Could you check a few things on this model? Use its own coordinates, in mm. A direction names the side the tool comes from. Round coordinates to 2 decimals unless told otherwise and drop trailing zeros. Loops run counter-clockwise (first coordinate to the right, second up) from the corner with the lowest first, then second, coordinate; pieces in that order, holes last.
from build123d import *

# Parameters (mm, degrees)
BOSS_EXTRUDE1_DEPTH           = 13
BOSS_EXTRUDE1_OTHER_WAY_DEPTH = 13
BOSS_EXTRUDE1_OTHER_WAY_TAPER = -0.2
SKETCH3_R                     = 8.5
BOSS_EXTRUDE2_DEPTH           = 2
CUT_EXTRUDE2_DEPTH            = 12.5
SKETCH2_R                     = 1.25
CUT_EXTRUDE1_DEPTH            = 15
CUT_EXTRUDE3_DEPTH            = 15


with BuildPart() as part:
    # Sketch1 → Boss-Extrude1 (new body)
    with BuildSketch(Plane.XY):
        with BuildLine():
            ThreePointArc((-6.053717866, -0.75), (6.1, 0), (-6.053717866, 0.75))
            Line((-6.053717866, 0.75), (-6.853717866, 0.5))
            Line((-6.853717866, 0.5), (-6.853717866, -0.5))
            Line((-6.853717866, -0.5), (-6.053717866, -0.75))
        make_face()
    extrude(amount=BOSS_EXTRUDE1_DEPTH)

    # Sketch1 → Boss-Extrude1 other way (add)
    with BuildSketch(Plane.XY):
        with BuildLine():
            ThreePointArc((-6.053717866, -0.75), (6.1, 0), (-6.053717866, 0.75))
            Line((-6.053717866, 0.75), (-6.853717866, 0.5))
            Line((-6.853717866, 0.5), (-6.853717866, -0.5))
            Line((-6.853717866, -0.5), (-6.053717866, -0.75))
        make_face()
    extrude(amount=-BOSS_EXTRUDE1_OTHER_WAY_DEPTH, taper=BOSS_EXTRUDE1_OTHER_WAY_TAPER)

    # Sketch3 → Boss-Extrude2 (add)
    with BuildSketch(Plane(origin=(0, 0, -13), x_dir=(-1, 0, 0), z_dir=(0, 0, -1))):
        Circle(SKETCH3_R)
    extrude(amount=BOSS_EXTRUDE2_DEPTH)

    # Sketch4 → Cut-Extrude2 (cut)
    with BuildSketch(Plane(origin=(0, 0, -15), x_dir=(-1, 0, 0), z_dir=(0, 0, -1))):
        with BuildLine():
            Line((2.5, 1.833030278), (2.5, -1.833030278))
            ThreePointArc((2.5, -1.833030278), (-3.1, 0), (2.5, 1.833030278))
        make_face()
    extrude(amount=-CUT_EXTRUDE2_DEPTH, mode=Mode.SUBTRACT)

    # Sketch2 → Cut-Extrude1 (cut)
    with BuildSketch(Plane.XY.offset(13)):
        Circle(SKETCH2_R)
    extrude(amount=-CUT_EXTRUDE1_DEPTH, mode=Mode.SUBTRACT)

    # Sketch5 → Cut-Extrude3 (cut)
    with BuildSketch(Plane.XY.offset(13)):
        with BuildLine():
            Line((-1.054239307, 0.67162451), (-5.182959865, 3.301909593))
            ThreePointArc((-5.182959865, 3.301909593), (-4.345438983, 4.345438983), (-3.301909593, 5.182959865))
            Line((-3.301909593, 5.182959865), (-0.67162451, 1.054239307))
            ThreePointArc((-0.67162451, 1.054239307), (-0.883883476, 0.883883476), (-1.054239307, 0.67162451))
        make_face()
        with BuildLine():
            Line((0.67162451, 1.054239307), (3.301909593, 5.182959865))
            ThreePointArc((3.301909593, 5.182959865), (4.345438983, 4.345438983), (5.182959865, 3.301909593))
            Line((5.182959865, 3.301909593), (1.054239307, 0.67162451))
            ThreePointArc((1.054239307, 0.67162451), (0.883883476, 0.883883476), (0.67162451, 1.054239307))
        make_face()
        with BuildLine():
            Line((1.054239307, -0.67162451), (5.182959865, -3.301909593))
            ThreePointArc((5.182959865, -3.301909593), (4.345438983, -4.345438983), (3.301909593, -5.182959865))
            Line((3.301909593, -5.182959865), (0.67162451, -1.054239307))
            ThreePointArc((0.67162451, -1.054239307), (0.883883476, -0.883883476), (1.054239307, -0.67162451))
        make_face()
        with BuildLine():
            Line((-0.67162451, -1.054239307), (-3.301909593, -5.182959865))
            ThreePointArc((-3.301909593, -5.182959865), (-4.345438983, -4.345438983), (-5.182959865, -3.301909593))
            Line((-5.182959865, -3.301909593), (-1.054239307, -0.67162451))
            ThreePointArc((-1.054239307, -0.67162451), (-0.883883476, -0.883883476), (-0.67162451, -1.054239307))
        make_face()
    extrude(amount=-CUT_EXTRUDE3_DEPTH, mode=Mode.SUBTRACT)


solid = part.part
Item 1: For faces 1 (the cylindrical face through (0, -6.1, 6.4)), 2 (the flat face through (-6.459, -0.623, 6.409)), 3 (the flat face through (-1.958, -3.074, 5.605)), which set-ups out of +Z, -Z, +X, -X, +Y, -Y let a thin tool reach every point of the face, with its end or its side?
Results list:
face 1: +Z, -Y
face 2: +Z, -X, -Y
face 3: +Z
Item 2: If I drill on line 1 along Y through (x, z) = (0, -11.5); line 2 along X through (y, z) = (2, 1.5); line 3 along X through (y, z) = (-1.5, 4.25), over which ranges is the centre line in solid material (lowest first)?
Results list:
line 1: y = -6.14 to -3.1, 3.1 to 6.14
line 2: x = -5.76 to -3.14, -1.27 to 1.27, 3.14 to 5.76
line 3: x = -5.91 to -2.35, -0.96 to 0.96, 2.35 to 5.91
Item 3: We'd pull the mould along Y, two halves only. Please class faces 4 (the flat face through (0, 4, 13)), 5 (the cylindrical face through (6.1, 0, 6.4)), 6 (the flat face through (0, 0, -2.5)), 7 (the cylindrical face through (3.1, -0.1, -8.8)): released by +Y, released by -Y, zero draft, split by the parting line, or undercut.
Results list:
face 4: zero draft
face 5: split by the parting line
face 6: undercut
face 7: undercut
Item 4: If we section it at B-B, the plane y = 7.5: Please give me the cut outline in (x, z), then the cut area to 3 significant figures.
Results list:
outline: (-4, -15) - (4, -15) - (4, -13) - (-4, -13) - close
area: 16.0 mm2
Item 5: Will these pins go through, and if not, where does the flat tip stop? pin 1 (3.5 mm diameter, centred on x = 0, y = 0, fed in from -Z); pin 2 (3 mm diameter, centred on y = 6, z = 4, fed in from -X); pin 3 (2 mm diameter, centred on x = -4.5, z = -0.5, fed in from +Y).
Results list:
pin 1: stops at z = -2.5
pin 2: stops at x = -3.28
pin 3: stops at y = 3.28
Item 6: If we section it at A-A, the plane z = 3.5: Please give me the cut outline in (x, y), then the cut area to 3 significant figures.
Results list:
outline: (-6.85, -0.5) - (-6.05, -0.75) arc R6.1 ccw to (-5.14, -3.28) - (-1.05, -0.67) arc R1.25 cw to (-1.05, 0.67) - (-5.14, 3.28) arc R6.1 ccw to (-6.05, 0.75) - (-6.85, 0.5) - close; (-3.28, -5.14) arc R6.1 ccw to (3.28, -5.14) - (0.67, -1.05) arc R1.25 cw to (-0.67, -1.05) - close; (-3.28, 5.14) - (-0.67, 1.05) arc R1.25 cw to (0.67, 1.05) - (3.28, 5.14) arc R6.1 ccw to start; (1.05, -0.67) - (5.14, -3.28) arc R6.1 ccw to (5.14, 3.28) - (1.05, 0.67) arc R1.25 cw to start
area: 81.8 mm2
Item 7: If we section it at C-C, the plane x = 7.25: Please give me the cut outline in (y, z), then the cut area to 3 significant figures.
Results list:
outline: (-4.44, -15) - (4.44, -15) - (4.44, -13) - (-4.44, -13) - close
area: 17.7 mm2
